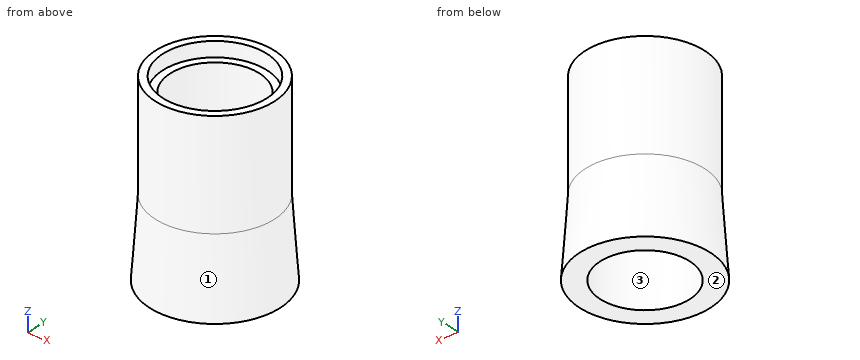
from build123d import *

# Parameters (mm, degrees)
SKETCH1_R           = 50.8
SKETCH1_R_2         = 38.1
BOSS_EXTRUDE1_DEPTH = 157.734
SKETCH2_R           = 38.1
SKETCH2_R_2         = 44.45
CUT_EXTRUDE1_DEPTH  = 12.7


with BuildPart() as part:
    # Sketch1 → Boss-Extrude1 (new body)
    with BuildSketch(Plane.XY):
        Circle(SKETCH1_R)
        Circle(SKETCH1_R_2, mode=Mode.SUBTRACT)
    extrude(amount=BOSS_EXTRUDE1_DEPTH)

    # Sketch2 → Cut-Extrude1 (cut)
    with BuildSketch(Plane.XY.offset(157.734)):
        Circle(SKETCH2_R)
        Circle(SKETCH2_R_2)
        Circle(SKETCH2_R, mode=Mode.SUBTRACT)
    extrude(amount=-CUT_EXTRUDE1_DEPTH, mode=Mode.SUBTRACT)

    # Sketch3 → Revolve1 (revolve)
    with BuildSketch(Plane(origin=(0, 0, 0), x_dir=(1, 0, 0), z_dir=(0, 1, 0))):
        Polygon((55.5625, 0), (50.8, -66.675), (50.8, 0), align=None)
    revolve(axis=Axis((0, 0, 0), (0, 0, 1)))


solid = part.part
Geometry: final body of the model. Coordinates: model frame, mm. Face numbers are marked on the shaded views. Coordinates: 2 decimals unless noted, no trailing zeros. Order: outer loops, then holes, each group sorted by start corner. A loop starts at its lowest first (then second) coordinate and runs counter-clockwise, first axis right, second up.
(1) Material intervals for probe 1 along Y at (x, z) = (0, 148); probe 2 along X at (y, z) = (30.5, 58); probe 3 along Y at (x, z) = (17.5, 17.5), sorted ascending.
(2) Section query D-D (z = 20). Return the cut outline in (x, y), plus the area to 3 significant figures.
(3) First-contact query: pin 1 (3 mm diameter, centred on x = -15, z = 88, fed in from +Y); pin 2 (10 mm diameter, centred on x = 42.5, y = 19, fed in from -Z); pin 3 (2 mm diameter, centred on y = -22.5, z = 66, fed in from +X); pin 4 (3 mm diameter, centred on y = -4.5, z = 97.5, fed in from +X). Flat tips, straight axial feed; report the tip coordinate or a pass-through.
(4) Draft query along Y for the marked faces 1, 2 and 3. Return one class per face: pulls with the +Y half, pulls with the -Y half, needs draft (parallel to the pull), parting line crosses it, or undercut.
(5) Section query C-C (z = 122.5). Return the cut outline in (x, y), plus the area to 3 significant figures.
Solution:
1. probe 1: y = -50.8 to -44.45, 44.45 to 50.8
1. probe 2: x = -41.4 to -22.83, 22.83 to 41.4
1. probe 3: y = -51.42 to -33.84, 33.84 to 51.42
2. outline: circle Ø108.27 at (0, 0); hole circle Ø76.2 at (0, 0)
2. area: 4,650 mm2
3. pin 1: stops at y = 48.97
3. pin 2: stops at z = 0
3. pin 3: stops at x = 46.09
3. pin 4: stops at x = 50.71
4. face 1: parting line crosses it
4. face 2: needs draft
4. face 3: undercut
5. outline: circle Ø101.6 at (0, 0); hole circle Ø76.2 at (0, 0)
5. area: 3,550 mm2
